Design review of the part built by this model. Coordinates are the model's own, in mm. A direction names the side the tool comes from. Round coordinates to 2 decimals unless told otherwise and drop trailing zeros. Order: outer loops, then holes, each group sorted by start corner. A loop starts at its lowest first (then second) coordinate and runs counter-clockwise, first axis right, second up. Notation, with made-up numbers: (-32.5, 6.25) - (-11.5, 6.25) arc R23 ccw to (-11.5, 28.25) - close; hole circle Ø8 at (73.5, 89). An arc over 180 degrees is marked (long way). Write item = value, one per line.
from build123d import *

# Parameters (mm, degrees)
SKETCH_1_R          = 32.5
EXTRUDE_1_DEPTH     = 36
SKETCH_2_R          = 38.5
EXTRUDE_2_DEPTH     = 82
SKETCH_3_R          = 41
EXTRUDE_3_DEPTH     = 12
SKETCH_4_R          = 35
EXTRUDE_4_DEPTH     = 76
SKETCH_5_R          = 32.5
EXTRUDE_5_DEPTH     = 64
SKETCH_6_R          = 31
EXTRUDE_6_DEPTH     = 50
SKETCH_7_R          = 27.5
EXTRUDE_7_DEPTH     = 82
FILLET_1_R          = 2
FILLET_2_R          = 1.6
CHAMFER_1_SIZE      = 2
CUT_EXTRUDE_1_DEPTH = 29
CUT_EXTRUDE_2_DEPTH = 20
SKETCH_10_R         = 3
CUT_EXTRUDE_3_DEPTH = 20


with BuildPart() as part:
    # 草图1 → 凸台-拉伸1 (new body)
    with BuildSketch(Plane.XY):
        Circle(SKETCH_1_R)
    extrude(amount=EXTRUDE_1_DEPTH)

    # 草图2 → 凸台-拉伸2 (add)
    with BuildSketch(Plane.XY.offset(36)):
        Circle(SKETCH_2_R)
    extrude(amount=EXTRUDE_2_DEPTH)

    # 草图3 → 凸台-拉伸3 (add)
    with BuildSketch(Plane.XY.offset(118)):
        Circle(SKETCH_3_R)
    extrude(amount=EXTRUDE_3_DEPTH)

    # 草图4 → 凸台-拉伸4 (add)
    with BuildSketch(Plane.XY.offset(130)):
        Circle(SKETCH_4_R)
    extrude(amount=EXTRUDE_4_DEPTH)

    # 草图5 → 凸台-拉伸5 (add)
    with BuildSketch(Plane.XY.offset(206)):
        Circle(SKETCH_5_R)
    extrude(amount=EXTRUDE_5_DEPTH)

    # 草图6 → 凸台-拉伸6 (add)
    with BuildSketch(Plane.XY.offset(270)):
        Circle(SKETCH_6_R)
    extrude(amount=EXTRUDE_6_DEPTH)

    # 草图7 → 凸台-拉伸7 (add)
    with BuildSketch(Plane.XY.offset(320)):
        Circle(SKETCH_7_R)
    extrude(amount=EXTRUDE_7_DEPTH)

    # 圆角1
    fillet_1_edges = [part.edges().sort_by_distance(p)[0] for p in [
        (-35, 0, 130),
        (-32.5, 0, 206),
    ]]
    fillet(fillet_1_edges, radius=FILLET_1_R)

    # 圆角2
    # the kernel refuses this fillet: 1.6 mm, written as the material it adds along each edge
    with BuildSketch(Plane(origin=(0, 0, 270), x_dir=(1, 0, 0), z_dir=(0, -1, 0))) as fillet_2_piece_1:
        with BuildLine():
            CenterArc((32.6, 1.596871942), FILLET_2_R, 180, 86.416678302)
            Line((31, 1.596871942), (30.968, 1.596871942))
            Line((30.968, 1.596871942), (30.968, 0))
            Line((30.968, 0), (31, -0.032))
            ThreePointArc((31, -0.032), (31.75, -0.032), (32.498, -0.031937439))
            Line((32.498, -0.031937439), (32.5, 0))
        make_face()
    revolve(axis=Axis((0, 0, 270), (0, 0, 1)))
    with BuildSketch(Plane(origin=(0, 0, 320), x_dir=(1, 0, 0), z_dir=(0, -1, 0))) as fillet_2_piece_2:
        with BuildLine():
            CenterArc((27.5 + FILLET_2_R, FILLET_2_R), FILLET_2_R, 180, 90)
            Line((27.5, FILLET_2_R), (27.5 - FILLET_2_R * 0.02, FILLET_2_R))
            Line((27.5 - FILLET_2_R * 0.02, FILLET_2_R), (27.5 - FILLET_2_R * 0.02, -FILLET_2_R * 0.02))
            Line((27.5 - FILLET_2_R * 0.02, -FILLET_2_R * 0.02), (27.5 + FILLET_2_R, -FILLET_2_R * 0.02))
            Line((27.5 + FILLET_2_R, -FILLET_2_R * 0.02), (27.5 + FILLET_2_R, 0))
        make_face()
    revolve(axis=Axis((0, 0, 320), (0, 0, 1)))

    # 倒角1
    chamfer_1_edges = [part.edges().sort_by_distance(p)[0] for p in [
        (-32.5, 0, 0),
        (-27.5, 0, 402),
    ]]
    chamfer(chamfer_1_edges, length=CHAMFER_1_SIZE)

    # 草图8 → 切除-拉伸1 (cut)
    with BuildSketch(Plane(origin=(27.5, 0, 0), x_dir=(0, 0, -1), z_dir=(1, 0, 0))):
        with BuildLine():
            Line((-189, 10), (-146, 10))
            ThreePointArc((-146, 10), (-136, 0), (-146, -10))
            Line((-146, -10), (-189, -10))
            ThreePointArc((-189, -10), (-199, 0), (-189, 10))
        make_face()
    extrude(amount=CUT_EXTRUDE_1_DEPTH, mode=Mode.SUBTRACT)

    # 草图9 → 切除-拉伸2 (cut)
    with BuildSketch(Plane(origin=(21.5, 0, 0), x_dir=(0, 0, -1), z_dir=(1, 0, 0))):
        with BuildLine():
            Line((-402, 8), (-334, 8))
            ThreePointArc((-334, 8), (-326, 0), (-334, -8))
            Line((-334, -8), (-402, -8))
            Line((-402, -8), (-402, 8))
        make_face()
    extrude(amount=CUT_EXTRUDE_2_DEPTH, mode=Mode.SUBTRACT)

    # 草图10 → 切除-拉伸3 (cut)
    with BuildSketch(Plane.XY.offset(402)):
        with Locations((0, 15)):
            Circle(SKETCH_10_R)
        with Locations((0, -15)):
            Circle(SKETCH_10_R)
    extrude(amount=-CUT_EXTRUDE_3_DEPTH, mode=Mode.SUBTRACT)


solid = part.part
Item 1: The part is to be moulded in two halves that separate along Z. For faces 1 (the face through (-9, -40, 124)), 2 (the face through (31, 0, 199)), 3 (the face through (-1, 0, 402)), say which applies: +Z half, -Z half, draft (parallel to the pull), parting line (faces both ways), or undercut.
Data:
face_1 = draft
face_2 = undercut
face_3 = +Z half
Item 2: Take a section at A-A, the plane z = 175. State the section outline as (x, y) points.
Data:
outline = (27.5, -10) - (27.5, 10) - (33.54, 10) arc R35 ccw (long way) to (33.54, -10) - close
Item 3: For line 1 along Y through (x, z) = (0, 389); line 2 along Z through (x, y) = (16, 26); line 3 along X through (y, z) = (6, 168.5), list the stretches that pass through material, from the lowest coordinate up. Write a range as [from, to].
Data:
line_1 = [-27.5, -18], [-12, 12], [18, 27.5]
line_2 = [0.03, 320]
line_3 = [-34.48, 27.5]
Item 4: Insertion check: P1, Ø4, axis at y = -30, z = 317.5, coming from the +X side; P2, Ø3, axis at y = -23, z = 44.5, coming from the -X side; P3, Ø3, axis at x = 31, z = 159.5, coming from the -Y side; P4, Ø9.5, axis at x = 0, y = 15, coming from the -Z side. Each pin has a flat end and moves straight along its axis. Give the tip position at first contact, or say it passes through.
Data:
P1 = 13.3
P2 = -31.94
P3 = -18.83
P4 = 0
Item 5: Take a section at B-B, the plane z = 283.5. State the section outline as (x, y) points, and give its area (3 significant figures).
Data:
outline = circle Ø62 at (0, 0)
area = 3,020 mm2
Item 6: For faces 4 (the face through (24, 0, 326)), 5 (the face through (-26, -20, 36)), 6 (the face through (-28, -21, 168)), list the 3-axis set-ups (+Z, -Z, +X, -X, +Y, -Y) from which the entire face can be reached by the end or side of a thin tool; tool diameter is ignored.
Data:
face_4 = +Z, +X
face_5 = -Z
face_6 = +Z
